Input: part model. Units: mm. Frame: model coordinates. A direction names the side the tool comes from. Coordinates: 2 decimals unless noted, no trailing zeros. Write each loop counter-clockwise with the first axis right and the second up, starting at its lowest first coordinate (ties: lowest second). Pieces come first, ordered by that corner, then holes. Notation, with made-up numbers: M 31,76 L 42,76 A10 ccw 42,88 Z; hole C -37.5,50.25 d11. An arc over 180 degrees is marked long. Answer as a JSON object with one key per item and string values. Group by question number.
Autodesk Inventor part; units mm, degrees
ref_plane "YZ Plane" through (0, 0, 0) normal (1, 0, 0) x (0, 1, 0)
ref_plane "XZ Plane" through (0, 0, 0) normal (0, 1, 0) x (-1, 0, 0)
ref_plane "XY Plane" through (0, 0, 0) normal (0, 0, 1) x (1, 0, 0)
sketch "Sketch1" plane through (0, 0, 0) normal (1, 0, 0) x (0, 1, 0)
  arc A0 (0, -12.7) -> (0, 12.7) centre (0, 0) ccw
  line L0 (0, -12.7) -> (-57.15, -12.7)
  line L1 (-57.15, -12.7) -> (-57.15, 12.7)
  line L2 (-57.15, 12.7) -> (0, 12.7)
  dimension "d0" = 25.4
  dimension "d1" = 57.15
extrude "Extrusion1" add sketch "Sketch1" against normal blind 111.76
sketch "Sketch2" plane through (0, -57.15, 12.7) normal (0, 0, 1) x (1, 0, 0)
  line L0 (0, 57.15) -> (0, 0)
  line L1 (0, 57.15) -> (-111.76, 57.15)
  line L2 (-111.76, 0) -> (-111.76, 57.15)
  line L3 (0, 0) -> (-111.76, 0)
  line L4 (-108.585, 3.175) -> (-108.585, 53.975)
  line L5 (-108.585, 53.975) -> (-3.175, 53.975)
  line L6 (-3.175, 53.975) -> (-3.175, 3.175)
  line L7 (-3.175, 3.175) -> (-108.585, 3.175)
  line L8 (-108.585, 53.975) -> (-108.585, 116.1509)
  line L9 (-108.585, 116.1509) -> (-5.0285, 113.469)
  line L10 (-3.175, 53.975) -> (-3.175, 108.1053)
  line L11 (-3.175, 108.1053) -> (-18.8552, 122.8908)
  point P0 (-8.9715, 113.5711)
  dimension "d4" = 3.175
extrude "Extrusion2" cut sketch "Sketch2" against normal blind 111.76 contours L10 L5 L8 L1 | L1 L8 L9 L11 L10 | L6 L7 L4 L5
sketch "Sketch3" plane through (0, 0, 0) normal (1, 0, 0) x (0, 0, -1)
  circle A0 centre (0, 0) radius 5.3975
  dimension "d7" = 10.795
sketch "Sketch4" plane through (-111.76, 0, 0) normal (-1, 0, 0) x (0, 0, 1)
  circle A0 centre (0, 0) radius 5.3975
  dimension "d8" = 10.795
extrude "Extrusion3" add sketch "Sketch4" along normal blind 3.175
fillet "Fillet1" radius 2.54 1 edges at (-114.935, 0, -5.3975)
extrude "Extrusion4" add sketch "Sketch3" along normal blind 3.175
fillet "Fillet2" radius 2.54 1 edges at (3.175, 0, 5.3975)
properties part number "box bot"
Q1. Pin query (flat end, axial travel): pin 1 Ø7.5 at (y, z) = (-17.5, -6) entering from -X; pin 2 Ø1.5 at (x, z) = (-17.5, -1) entering from +Y (3 decimals); pin 3 Ø2 at (y, z) = (-7.5, 9) entering from +X. Return the tip coordinate at first contact, or that it passes through.
Q2. Access query for faces 1 (the cylindrical face through (-112.073, -3.648, -3.978)), 2 (the flat face through (-3.175, -21, 0)), 3 (the flat face through (-55, -57.15, 0)). Directions: +Z, -Z, +X, -X, +Y, -Y. A direction counts if a zero-diameter tool reaches every point of the face in a straight line with its end or side. Return the directions, or none.
Q3. Section A-A, the plane y = -48.5. Return the cut outline in (x, z) (3 decimals).
Q4. Section C-C, the plane x = -106.5. Return the cut outline in (y, z) (3 decimals), and give its area (3 significant figures).
Q5. Section D-D, the plane y = 7.5. Return the cut outline in (x, z) (3 decimals).
Q6. Draft query along X for faces 4 (the cylindrical face through (0.313, -3.648, 3.978)), 5 (the flat face through (-108.585, -21, 0)), 6 (the flat face through (0, -23, 0)). Return one class per face: released by +X, released by -X, zero draft, split by the parting line, or undercut.
Q7. Line query: line 1 (X direction, y = -39.5, z = -6.75) (3 decimals); line 2 (Y direction, x = -101.5, z = -5.75) (3 decimals); line 3 (X direction, y = -3, z = -3.5) (3 decimals). Output: solid intervals per line, ascending. Write a range as from..to.
Filled in:
{
 "1": {"pin 1": "x = -111.76", "pin 2": "y = -53.975", "pin 3": "x = 0"},
 "2": {"face 1": "-X", "face 2": "+Z, -Z, +Y", "face 3": "+Z, -Z, +X, -X, -Y"},
 "3": {"outline": "M -111.76,-12.7 L -108.585,-12.7 L -108.585,12.7 L -111.76,12.7 Z; M -3.175,-12.7 L 0,-12.7 L 0,12.7 L -3.175,12.7 Z"},
 "4": {"outline": "M -57.15,-12.7 L -53.975,-12.7 L -53.975,12.7 L -57.15,12.7 Z", "area": "80.6 mm^2"},
 "5": {"outline": "M -111.76,-10.249 L -108.585,-10.249 L -108.585,10.249 L -111.76,10.249 Z; M -3.175,-10.249 L 0,-10.249 L 0,10.249 L -3.175,10.249 Z"},
 "6": {"face 4": "zero draft", "face 5": "undercut", "face 6": "released by +X"},
 "7": {"line 1": "-111.76..-108.585, -3.175..0", "line 2": "-57.15..-53.975", "line 3": "-114.234..-108.585, -3.175..2.474"}
}
